Geometry check sheet. Reference: the model listing, model coordinates, mm. A direction names the side the tool comes from. Coordinates: 2 decimals unless noted, no trailing zeros. Order: outer loops, then holes, each group sorted by start corner. A loop starts at its lowest first (then second) coordinate and runs counter-clockwise, first axis right, second up. Notation, with made-up numbers: (13, 85.5) - (54, 85.5) arc R30 ccw to (54, 124.5) - close; hole circle Ø3 at (43, -26.75). An arc over 180 degrees is marked (long way). Return JSON: item names as keys, results as strings. Group by question number.
Item 1: Gauge pin test, flat ends, axial feed: pin 1 (1.5 mm diameter, centred on y = 6.5, z = -2, fed in from +X); pin 2 (2.5 mm diameter, centred on x = 6.5, z = -3.5, fed in from +Y); pin 3 (3 mm diameter, centred on x = 5.75, z = -2.55, fed in from -Y); pin 4 (1.6 mm diameter, centred on y = 5.7, z = -2.55, fed in from -X). Record the tip position at first contact, or that the pin passes through.
Item 2: Tool access check on faces 5 (the cylindrical face through (2.307, 7.652, -2.116)), 6 (the flat face through (6, 3, -1)), 7 (the flat face through (3, 2, 0)). Record the directions out of +Z, -Z, +X, -X, +Y, -Y that give a thin tool (end or side, any length) a straight path to the whole face; none if there is none.
Item 3: Draft check along X on faces 1 (the flat face through (1, 8.25, -3)), 2 (the cylindrical face through (5.45, 2.29, -3.5)), 3 (the cylindrical face through (7.7, 0.5, -2.1)), 4 (the flat face through (2.8, 4, -1)). Enter one of: pulls with the +X half, pulls with the -X half, needs draft (parallel to the pull), parting line crosses it, or undercut.
Item 4: Section check B-B on x = 2. Enter the section's corners in (y, z).
Item 5: Section check D-D on y = 2.5. Enter the section's corners in (x, z).
Item 6: Scan lines: probe 1 along Z at (x, y) = (0.45, 5.7); probe 2 along Z at (x, y) = (2.25, 5.7); probe 3 along X at (y, z) = (4, -4.9). Record each from-to range of solid material in increasing order.
Item 7: Section check A-A on y = 5.7. Enter the section's corners in (x, z).
Item 8: Section check C-C on z = -2.55. Give the number of separate pieces and of enclosed holes in the cut face, then the cut area to 3 significant figures.
from build123d import *

# Parameters (mm, degrees)
ESQUISSE1_W        = 8.3
ESQUISSE1_H        = 5.1
BOSS_EXTRU_1_DEPTH = 3
ESQUISSE2_W        = 2.8
ESQUISSE2_H        = 5.1
BOSS_EXTRU_2_DEPTH = 5.25


with BuildPart() as part:
    # Esquisse1 → Boss.-Extru.1 (new body)
    with BuildSketch(Plane(origin=(0, 0, 0), x_dir=(1, 0, 0), z_dir=(0, 1, 0))):
        with Locations((4.15, 2.55)):
            Rectangle(ESQUISSE1_W, ESQUISSE1_H)
    extrude(amount=BOSS_EXTRU_1_DEPTH)

    # Esquisse2 → Boss.-Extru.2 (add)
    with BuildSketch(Plane(origin=(0, 3, 0), x_dir=(1, 0, 0), z_dir=(0, 1, 0))):
        with Locations((1.4, 2.55)):
            Rectangle(ESQUISSE2_W, ESQUISSE2_H)
    extrude(amount=BOSS_EXTRU_2_DEPTH)

    # Esquisse6 → Perçage1 (revolve, cut)
    with BuildSketch(Plane(origin=(2.8, 5.7, -2.55), x_dir=(0, 0, -1), z_dir=(0, 1, 0))):
        Polygon((0, 0), (0, 3.400860619), (1, 2.8), (1, 1.600860619), (2, 1), (2, 0), align=None)
    revolve(axis=Axis((8.930023899, 5.7, -2.55), (-1, 0, 0)), mode=Mode.SUBTRACT)

    # Esquisse9 → Perçage2 (revolve, cut)
    with BuildSketch(Plane(origin=(5.750237397, 0, -2.547317036), x_dir=(0, 0, -1), z_dir=(1, 0, 0))):
        Polygon((0, 0), (0, 10.600860619), (1, 10), (1, 1.600860619), (2, 1), (2, 0), align=None)
    revolve(axis=Axis((5.750237397, -6.130023899, -2.547317036), (0, 1, 0)), mode=Mode.SUBTRACT)


solid = part.part
Computed:
{
 "1": {"pin 1": "stops at x = 1.63", "pin 2": "stops at y = 3", "pin 3": "stops at y = 1.3", "pin 4": "passes through"},
 "2": {"face 5": "+X", "face 6": "+Z, -Z, +X, +Y", "face 7": "+Z, +X, -X, +Y, -Y"},
 "3": {"face 1": "needs draft", "face 2": "undercut", "face 3": "undercut", "face 4": "pulls with the +X half"},
 "4": {"outline": "(0, -5.1) - (8.25, -5.1) - (8.25, 0) - (0, 0) - close; hole circle Ø4 at (5.7, -2.55)"},
 "5": {"outline": "(0, -5.1) - (8.3, -5.1) - (8.3, 0) - (0, 0) - close; hole circle Ø2 at (5.75, -2.55)"},
 "6": {"probe 1": "z = -5.1 to -3.55, -1.55 to 0", "probe 2": "z = -5.1 to -4.55, -0.55 to 0", "probe 3": "x = 0 to 2.8"},
 "7": {"outline": "(0, -5.1) - (2.8, -5.1) - (2.8, -4.55) - (1.8, -4.55) - (1.2, -3.55) - (0, -3.55) - close; (0, -1.55) - (1.2, -1.55) - (1.8, -0.55) - (2.8, -0.55) - (2.8, 0) - (0, 0) - close"},
 "8": {"separate pieces": "3", "enclosed holes": "0", "area": "22.8 mm²"}
}
